Read the model definition and answer for the solid it produces. Units are mm, in the model's axes. Face numbers are marked on the shaded views. Round coordinates to 2 decimals unless told otherwise and drop trailing zeros. Order: outer loops, then holes, each group sorted by start corner. A loop starts at its lowest first (then second) coordinate and runs counter-clockwise, first axis right, second up. Notation, with made-up numbers: (56.25, 14.5) - (68.25, 14.5) arc R24 ccw to (68.25, 40.5) - close; hole circle Ø8 at (60, 27.5). An arc over 180 degrees is marked (long way). Answer as a JSON object with one key per item and string values. Group by question number.
Q1. The mould has two halves that part along X. Classify the marked faces 1, 2 and 3: pulls with the +X half, pulls with the -X half, needs draft (parallel to the pull), parting line crosses it, or undercut.
Q2. Given pin 1 Ø1.9 at (y, z) = (37, 22.5) entering from -X; pin 2 Ø1.1 at (y, z) = (22, -23) entering from +X; pin 3 Ø1.3 at (y, z) = (19, 18) entering from -X, each flat-ended and moving along its own axis, determine where each tip first touches the part or whether it passes through.
Q3. Consider line 1 (Z direction, x = 4.5, y = 29); line 2 (X direction, y = 37.5, z = 18); line 3 (Z direction, x = -2, y = 3.5) (3 decimals). Determine where each line is inside the solid, lowest interval first.
Q4. A cutting plane is placed at B-B on z = -3.5. Determine the outline of the cut face in (x, y).
Q5. A cutting plane is placed at A-A on y = 16.5. Determine the outline of the cut face in (x, z) (3 decimals), and give its area (3 significant figures).
Q6. A cutting plane is placed at C-C on x = -6.5. Determine the outline of the cut face in (y, z).
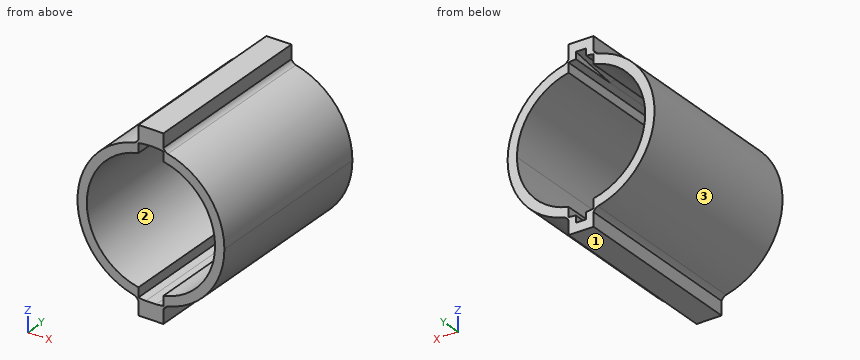
```python
from build123d import *

# Parameters (mm, degrees)
BOSS_EXTRUDE1_DEPTH     = 50
BOSS_EXTRUDE2_DEPTH     = 2.8
CUT_EXTRUDE1_DEPTH      = 60.094773246
CUT_EXTRUDE1_DEPTH_BACK = 60.094773246


with BuildPart() as part:
    # Sketch1 → Boss-Extrude1 (new body)
    with BuildSketch(Plane(origin=(0, 0, 0), x_dir=(1, 0, 0), z_dir=(0, 1, 0))):
        with BuildLine():
            Line((3.4, 20.590136136), (3.4, 19.708881247))
            ThreePointArc((3.4, 19.708881247), (4.001170568, 19.595678965), (4.598597833, 19.464143905))
            ThreePointArc((4.598597833, 19.464143905), (3.888587722, 19.909290009), (3.4, 20.590136136))
        make_face()
        with BuildLine():
            ThreePointArc((-4.598597833, 19.464143905), (-4.001170568, 19.595678965), (-3.4, 19.708881247))
            Line((-3.4, 19.708881247), (-3.4, 20.590136136))
            ThreePointArc((-3.4, 20.590136136), (-3.888587722, 19.909290009), (-4.598597833, 19.464143905))
        make_face()
        with BuildLine():
            Line((-1.4, 19.950939827), (-1.4, 21.835))
            Line((-1.4, 21.835), (1.4, 21.835))
            Line((1.4, 21.835), (1.4, 19.950939827))
            ThreePointArc((1.4, 19.950939827), (2.403049748, 19.855108962), (3.4, 19.708881247))
            Line((3.4, 19.708881247), (3.4, 20.590136136))
            Line((3.4, 20.590136136), (3.4, 24.335))
            Line((3.4, 24.335), (-3.4, 24.335))
            Line((-3.4, 24.335), (-3.4, 20.590136136))
            Line((-3.4, 20.590136136), (-3.4, 19.708881247))
            ThreePointArc((-3.4, 19.708881247), (-2.403049748, 19.855108962), (-1.4, 19.950939827))
        make_face()
        with BuildLine():
            Line((-3.4, 17.125758377), (-3.4, 19.708881247))
            ThreePointArc((-3.4, 19.708881247), (-4.001170568, 19.595678965), (-4.598597833, 19.464143905))
            ThreePointArc((-4.598597833, 19.464143905), (-20, 0), (-4.598597833, -19.464143905))
            ThreePointArc((-4.598597833, -19.464143905), (-4.001170568, -19.595678965), (-3.4, -19.708881247))
            Line((-3.4, -19.708881247), (-3.4, -17.125758377))
            ThreePointArc((-3.4, -17.125758377), (-17.46, 0), (-3.4, 17.125758377))
        make_face()
        with BuildLine():
            ThreePointArc((4.598597833, 19.464143905), (4.001170568, 19.595678965), (3.4, 19.708881247))
            Line((3.4, 19.708881247), (3.4, 17.125758377))
            ThreePointArc((3.4, 17.125758377), (13.494732306, 11.078980097), (17.46, 0))
            ThreePointArc((17.46, 0), (13.494732306, -11.078980097), (3.4, -17.125758377))
            Line((3.4, -17.125758377), (3.4, -19.708881247))
            ThreePointArc((3.4, -19.708881247), (4.001170568, -19.595678965), (4.598597833, -19.464143905))
            ThreePointArc((4.598597833, -19.464143905), (15.683940141, -12.410238582), (20, 0))
            ThreePointArc((20, 0), (15.683940141, 12.410238582), (4.598597833, 19.464143905))
        make_face()
        with BuildLine():
            ThreePointArc((4.598597833, -19.464143905), (4.001170568, -19.595678965), (3.4, -19.708881247))
            Line((3.4, -19.708881247), (3.4, -20.590136136))
            ThreePointArc((3.4, -20.590136136), (3.888587722, -19.909290009), (4.598597833, -19.464143905))
        make_face()
        with BuildLine():
            ThreePointArc((-3.4, -19.708881247), (-4.001170568, -19.595678965), (-4.598597833, -19.464143905))
            ThreePointArc((-4.598597833, -19.464143905), (-3.888587722, -19.909290009), (-3.4, -20.590136136))
            Line((-3.4, -20.590136136), (-3.4, -19.708881247))
        make_face()
        with BuildLine():
            Line((-1.4, -21.835), (-1.4, -19.950939827))
            ThreePointArc((-1.4, -19.950939827), (-2.403049748, -19.855108962), (-3.4, -19.708881247))
            Line((-3.4, -19.708881247), (-3.4, -20.590136136))
            Line((-3.4, -20.590136136), (-3.4, -24.335))
            Line((-3.4, -24.335), (3.4, -24.335))
            Line((3.4, -24.335), (3.4, -20.590136136))
            Line((3.4, -20.590136136), (3.4, -19.708881247))
            ThreePointArc((3.4, -19.708881247), (2.403049748, -19.855108962), (1.4, -19.950939827))
            Line((1.4, -19.950939827), (1.4, -21.835))
            Line((1.4, -21.835), (-1.4, -21.835))
        make_face()
    extrude(amount=BOSS_EXTRUDE1_DEPTH)

    # Sketch2 → Boss-Extrude2 (add)
    with BuildSketch(Plane(origin=(-1.4, 0, 0), x_dir=(0, 0, -1), z_dir=(1, 0, 0))):
        Polygon((21.835, 0), (21.835, 50), (19.950939827, 36.594215293), (19.950939827, 0), align=None)
        Polygon((-21.835, 50), (-21.835, 0), (-14.807958265, 0), align=None)
    extrude(amount=BOSS_EXTRUDE2_DEPTH)

    # Sketch3 → Cut-Extrude1 (cut, two sides: drawn at the far end of the back side and taken through both)
    with BuildSketch(Plane.XZ.offset(-CUT_EXTRUDE1_DEPTH_BACK)):
        with BuildLine():
            ThreePointArc((1.4, 19.950939827), (0, 20), (-1.4, 19.950939827))
            Line((-1.4, 19.950939827), (-1.4, 14.807958265))
            Line((-1.4, 14.807958265), (1.4, 14.807958265))
            Line((1.4, 14.807958265), (1.4, 19.950939827))
        make_face()
    extrude(amount=CUT_EXTRUDE1_DEPTH + CUT_EXTRUDE1_DEPTH_BACK, mode=Mode.SUBTRACT)


solid = part.part
```
Result set:
{
 "1": {"face 1": "needs draft", "face 2": "undercut", "face 3": "pulls with the -X half"},
 "2": {"pin 1": "stops at x = -3.4", "pin 2": "stops at x = 3.4", "pin 3": "stops at x = -9.95"},
 "3": {"line 1": "z = -19.5 to -16.87, 16.87 to 19.5", "line 2": "x = -8.72 to -3.4, 3.4 to 8.72", "line 3": "z = -24.335 to -19.9, 19.9 to 24.335"},
 "4": {"outline": "(-19.69, 0) - (-17.11, 0) - (-17.11, 50) - (-19.69, 50) - close; (17.11, 0) - (19.69, 0) - (19.69, 50) - (17.11, 50) - close"},
 "5": {"outline": "(-4.599, -19.464) arc R2.172 cw to (-3.4, -20.59) - (-3.4, -24.335) - (3.4, -24.335) - (3.4, -20.59) arc R2.172 cw to (4.599, -19.464) arc R20 ccw to (4.599, 19.464) arc R2.172 cw to (3.4, 20.59) - (3.4, 24.335) - (-3.4, 24.335) - (-3.4, 20.59) arc R2.172 cw to (-4.599, 19.464) arc R20 ccw to start; hole (-3.4, -19.709) arc R20 ccw to (-1.4, -19.951) - (1.4, -19.951) arc R20 ccw to (3.4, -19.709) - (3.4, -17.126) arc R17.46 ccw to (3.4, 17.126) - (3.4, 19.709) arc R20 ccw to (-3.4, 19.709) - (-3.4, 17.126) arc R17.46 ccw to (-3.4, -17.126) - close", "area": "326 mm²"},
 "6": {"outline": "(0, -18.91) - (50, -18.91) - (50, -16.2) - (0, -16.2) - close; (0, 16.2) - (50, 16.2) - (50, 18.91) - (0, 18.91) - close"}
}
